Part model, mm, in its own coordinate system. Face numbers are marked on the shaded views. A direction names the side the tool comes from. Round coordinates to 2 decimals unless told otherwise and drop trailing zeros. Write each loop counter-clockwise with the first axis right and the second up, starting at its lowest first coordinate (ties: lowest second). Pieces come first, ordered by that corner, then holes.
Autodesk Inventor part; units mm, degrees
ref_plane "YZ Plane" through (0, 0, 0) normal (1, 0, 0) x (0, 1, 0)
ref_plane "XZ Plane" through (0, 0, 0) normal (0, 1, 0) x (-1, 0, 0)
ref_plane "XY Plane" through (0, 0, 0) normal (0, 0, 1) x (1, 0, 0)
sketch "Sketch1" plane through (0, 0, 0) normal (0, 1, 0) x (-1, 0, 0)
  line L0 (-25.5, 57.5) -> (25.5, 57.5)
  line L1 (25.5, 57.5) -> (25.5, -57.5)
  line L2 (25.5, -57.5) -> (-25.5, -57.5)
  line L3 (-25.5, -57.5) -> (-25.5, 57.5)
  line L4 (-25.5, 57.5) -> (25.5, -57.5) construction
  line L5 (25.5, 57.5) -> (-25.5, -57.5) construction
  point P0 (0, 0)
  dimension "d0" = 51
  dimension "d1" = 115
extrude "Extrusion1" add sketch "Sketch1" along normal blind 33
sketch "Sketch2" plane through (-25.5, 0, 57.5) normal (0, 0, 1) x (1, 0, 0)
  circle A0 centre (10.5, 16.5) radius 4.875
  line L0 (0, 0) -> (0, 33)
  point P0 (25.5, 0)
  point P1 (0, 16.5)
  dimension "d4" = 10.5
  dimension "d5" = 9.75
extrude "Extrusion2" add sketch "Sketch2" along normal blind 13.4
properties part number "Power brick"
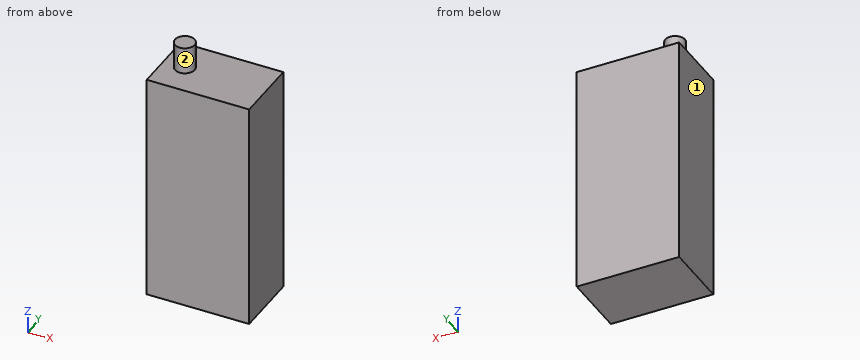
Q1. Cut at C-C on y = 4. Write the cut outline in (x, z), plus the area to 4 significant figures.
Values follow:
outline: (-25.5, -57.5) - (25.5, -57.5) - (25.5, 57.5) - (-25.5, 57.5) - close
area: 5,865 mm2
Q2. Which spindle directions (+Z, -Z, +X, -X, +Y, -Y) get a long thin tool onto all of the face, cutting with end or side? Do the marked faces 1 and 2. Say none if no direction does.
Values follow:
face 1: +Z, -Z, -X, +Y, -Y
face 2: +Z
Q3. Cut at A-A on x = -15. Write the cut outline in (y, z) (3 decimals), plus the area to 3 significant figures.
Values follow:
outline: (0, -57.5) - (33, -57.5) - (33, 57.5) - (21.375, 57.5) - (21.375, 70.9) - (11.625, 70.9) - (11.625, 57.5) - (0, 57.5) - close
area: 3,930 mm2
Q4. Wall check: L1, parallel to Z at x = 4, y = 16. Give the ranges that are in metal, low to high.
Values follow:
L1: z = -57.5 to 57.5
Q5. Drop a flat-ended pin along its axis: pin 1 (10 mm diameter, centred on x = -4, y = 13, fed in from +Z). Give the stop position or say it passes through.
Values follow:
pin 1: stops at z = 57.5
Q6. Cut at D-D on x = 0. Write the cut outline in (y, z), plus the area to 4 significant figures.
Values follow:
outline: (0, -57.5) - (33, -57.5) - (33, 57.5) - (0, 57.5) - close
area: 3,795 mm2
Q7. Cut at B-B on y = 16.5. Write the cut outline in (x, z) (3 decimals).
Values follow:
outline: (-25.5, -57.5) - (25.5, -57.5) - (25.5, 57.5) - (-10.125, 57.5) - (-10.125, 70.9) - (-19.875, 70.9) - (-19.875, 57.5) - (-25.5, 57.5) - close
